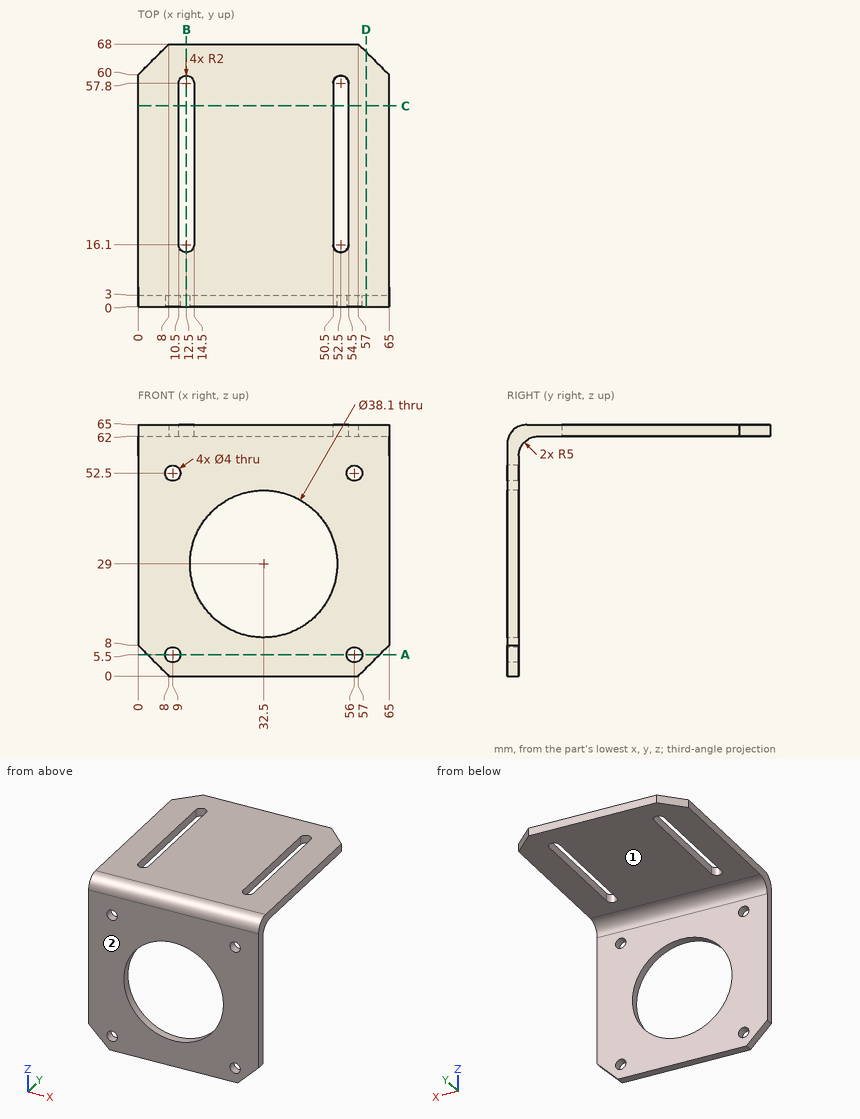
Geometry check sheet. Reference: drawing and pictorial views, mm from the part's lowest x, y, z. A direction names the side the tool comes from. Round coordinates to 2 decimals unless told otherwise and drop trailing zeros. Order: outer loops, then holes, each group sorted by start corner. A loop starts at its lowest first (then second) coordinate and runs counter-clockwise, first axis right, second up.
Q1. Set-up check for the marked faces 1 and 2: record each of +Z, -Z, +X, -X, +Y, -Y from which the full face is reachable in a straight line by a thin tool's end or side.
Filled sheet:
face 1: -Z, +X, -X, +Y
face 2: +Z, -Z, +X, -X, -Y
Q2. Cross-section at D-D, the plane x = 59. Enter the section's corners in (y, z).
Filled sheet:
outline: (0, 2) - (3, 2) - (3, 57) arc R5 cw to (8, 62) - (66, 62) - (66, 65) - (5, 65) arc R5 ccw to (0, 60) - close
Q3. Cross-section at A-A, the plane z = 5.5. Enter the section's corners in (x, y).
Filled sheet:
outline: (2.5, 0) - (7, 0) - (7, 3) - (2.5, 3) - close; (11, 0) - (54, 0) - (54, 3) - (11, 3) - close; (58, 0) - (62.5, 0) - (62.5, 3) - (58, 3) - close
Q4. Scan lines: L1, parallel to Y at x = 10.5, z = 33; L2, parallel to Z at x = 55.5, y = 25; L3, parallel to Y at x = 29.5, z = 61. Record each from-to range of solid material in increasing order.
Filled sheet:
L1: y = 0 to 3
L2: z = 62 to 65
L3: y = 0.1 to 5
Q5. Cross-section at B-B, the plane x = 12.5. Enter the section's corners in (y, z).
Filled sheet:
outline: (0, 0) - (3, 0) - (3, 57) arc R5 cw to (8, 62) - (14.1, 62) - (14.1, 65) - (5, 65) arc R5 ccw to (0, 60) - close; (59.8, 62) - (68, 62) - (68, 65) - (59.8, 65) - close
Q6. Depth check by flat-ended pin: P1, Ø23, axis at x = 32.5, z = 29, coming from the +Y side; P2, Ø3, axis at x = 56.5, y = 34, coming from the -Z side; P3, Ø5, axis at x = 9, z = 52.5, coming from the +Y side; P4, Ø10, axis at x = 23, z = 55, coming from the +Y side. Enter the tip coordinate at first touch or a pass-through.
Filled sheet:
P1: passes through
P2: stops at z = 62
P3: stops at y = 3
P4: stops at y = 4
Q7. Cross-section at C-C, the plane y = 52. Enter the section's corners in (x, z), plus the area to 3 significant figures.
Filled sheet:
outline: (0, 62) - (10.5, 62) - (10.5, 65) - (0, 65) - close; (14.5, 62) - (50.5, 62) - (50.5, 65) - (14.5, 65) - close; (54.5, 62) - (65, 62) - (65, 65) - (54.5, 65) - close
area: 171 mm2
